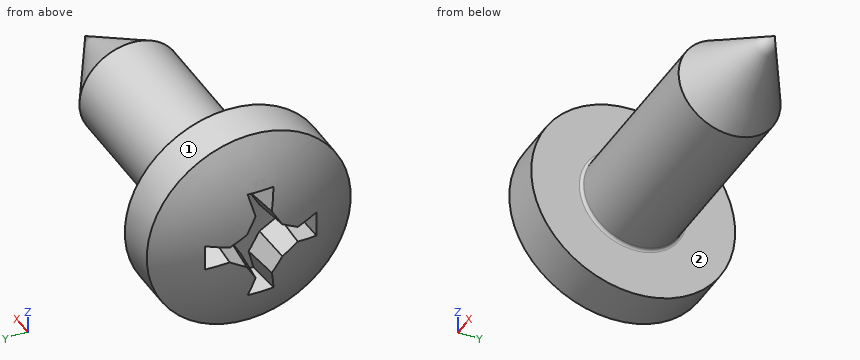
from build123d import *

# Parameters (mm, degrees)
CHAMFER1_SIZE      = 0.35
CHAMFER1_SIZE2     = 0.606217783
CUT_EXTRUDE1_DEPTH = 1.4
CUT_EXTRUDE1_TAPER = 6
FILLET1_R          = 0.1


with BuildPart() as part:
    # Sketch1 → Revolve1 (revolve)
    with BuildSketch(Plane.XY, mode=Mode.PRIVATE) as revolve1_sk:
        with BuildLine():
            Line((0, 3.5), (-1.473397172, 3.5))
            ThreePointArc((-1.473397172, 3.5), (-2.311408891, 1.838425545), (-2.6, 0))
            Line((-2.6, 0), (9.5, 0))
            Line((9.5, 0), (9.5, 1.75))
            Line((9.5, 1.75), (0, 1.75))
            Line((0, 1.75), (0, 3.5))
        make_face()
    revolve(revolve1_sk.sketch.rotate(Axis((0, 0, 0), (1, 0, 0)), 90), axis=Axis((0, 0, 0), (1, 0, 0)))

    # Chamfer1
    chamfer1_edges = [part.edges().sort_by_distance(p)[0] for p in [
        (9.5, 0, -1.75),
    ]]
    chamfer1_side = [part.faces().sort_by_distance(p)[0] for p in [
        (9.5, 0, 0),
    ]]
    chamfer(chamfer1_edges, length=CHAMFER1_SIZE, length2=CHAMFER1_SIZE2, reference=chamfer1_side[0])

    # Sketch2 → EndCone (revolve, cut)
    with BuildSketch(Plane.XY, mode=Mode.PRIVATE) as endcone_sk:
        Polygon((9.5, 0), (6.468911087, 1.75), (6.468911087, 1.85), (9.6, 1.85), (9.6, 0), align=None)
    revolve(endcone_sk.sketch.rotate(Axis((0, 0, 0), (1, 0, 0)), 90), axis=Axis((0, 0, 0), (1, 0, 0)), mode=Mode.SUBTRACT)

    # Sketch3 → Cut-Extrude1 (cut)
    with BuildSketch(Plane(origin=(-2.6, 0, 0), x_dir=(0, 0, -1), z_dir=(1, 0, 0))):
        Polygon((-0.4875, 1.95), (-0.2925, 1.17), (-0.613687292, 0.613687292), (-1.17, 0.2925), (-1.95, 0.4875), (-1.95, -0.4875), (-1.17, -0.2925), (-0.613687292, -0.613687292), (-0.2925, -1.17), (-0.4875, -1.95), (0.4875, -1.95), (0.2925, -1.17), (0.613687292, -0.613687292), (1.17, -0.2925), (1.95, -0.4875), (1.95, 0.4875), (1.17, 0.2925), (0.613687292, 0.613687292), (0.2925, 1.17), (0.4875, 1.95), align=None)
    extrude(amount=CUT_EXTRUDE1_DEPTH, taper=CUT_EXTRUDE1_TAPER, mode=Mode.SUBTRACT)

    # Fillet1
    fillet1_edges = [part.edges().sort_by_distance(p)[0] for p in [
        (0, 0, -1.75),
    ]]
    fillet(fillet1_edges, radius=FILLET1_R)


solid = part.part
Source: CAD feature listing. Evaluate the final solid. Frame: model axes, mm. Face numbers are marked on the shaded views. A direction names the side the tool comes from. Round coordinates to 2 decimals unless told otherwise and drop trailing zeros. Write each loop counter-clockwise with the first axis right and the second up, starting at its lowest first coordinate (ties: lowest second). Pieces come first, ordered by that corner, then holes. Notation, with made-up numbers: M 62,73.5 L 98,73.5 A20 cw 98,91.5 Z; hole C 58.5,30 d2. An arc over 180 degrees is marked long. One line per item, written item: value. Start each with the question number.
Item 1: Section query A-A (x = 5). Return the cut outline in (y, z), plus the area to 3 significant figures.
Item 2: Section query B-B (y = 2.5). Return the cut outline in (x, z).
Item 3: Pin query (flat end, axial travel): pin 1 (2 mm diameter, centred on y = 1.5, z = -2, fed in from -X); pin 2 (1 mm diameter, centred on x = 2.5, y = -1, fed in from +Z); pin 3 (3 mm diameter, centred on y = 1.5, z = 2, fed in from +X). Return the tip coordinate at first contact, or that it passes through.
Item 4: Ray query, L1, parallel to Y at x = 5.5, z = 0; L2, parallel to Y at x = -2, z = -0.5; L3, parallel to Z at x = 1.5, y = 0.75. Return the intervals inside material, ascending. Write a range as from..to.
Item 5: Set-up query: the marked faces 1 and 2. Return all of +Z, -Z, +X, -X, +Y, -Y with unobstructed straight access to the full face (end or side cutting, diameter ignored); none if empty.
Item 6: Section query C-C (z = 3.25). Return the cut outline in (x, y).
Result set:
1. outline: C 0,0 d3.5
1. area: 9.62 mm²
2. outline: M -1.47,-2.45 L 0,-2.45 L 0,2.45 L -1.47,2.45 A5.45 ccw Z
3. pin 1: stops at x = -2.41
3. pin 2: stops at z = 1.68
3. pin 3: stops at x = 7.77
4. L1: y = -1.75..1.75
4. L2: y = -2.57..-0.68, 0.68..2.57
4. L3: z = -1.58..1.58
5. face 1: +X, -X
5. face 2: +X
6. outline: M -1.47,-1.3 L 0,-1.3 L 0,1.3 L -1.47,1.3 A5.04 ccw Z
